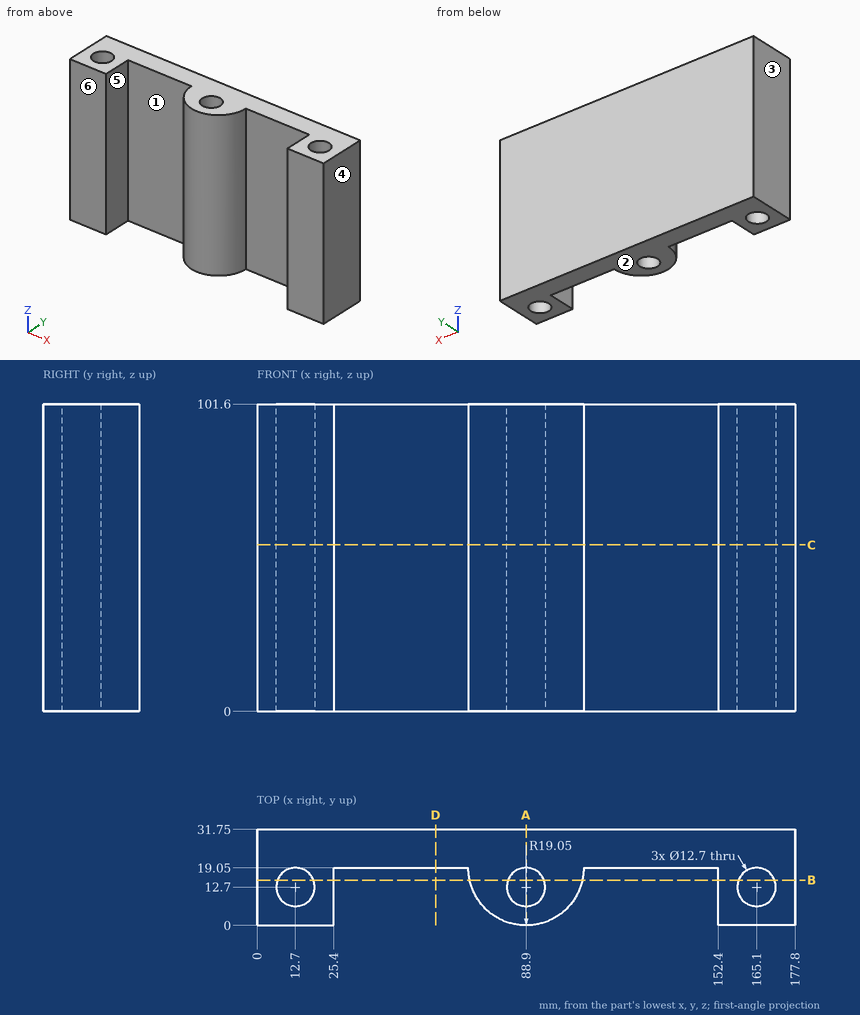
Source: three-view drawing plus pictorial views. Frame: mm from the lowest corner of the part. A direction names the side the tool comes from. Coordinates: 2 decimals unless noted, no trailing zeros. Order: outer loops, then holes, each group sorted by start corner. A loop starts at its lowest first (then second) coordinate and runs counter-clockwise, first axis right, second up. Notation, with made-up numbers: M 67.25,-34 L 100.25,-34 A30 ccw 100.25,4 Z; hole C 31.25,81 d2. An arc over 180 degrees is marked long. One line per question, with ' | ' between items.
Item 1: Section A-A (x = 88.9). Output: boundary loops of the cut face in (y, z).
Geometry results:
outline: M 0,0 L 6.35,0 L 6.35,101.6 L 0,101.6 Z; M 19.05,0 L 31.75,0 L 31.75,101.6 L 19.05,101.6 Z
Item 2: Ray query, line 1 along Y through (x, z) = (12.7, 45); line 2 along X through (y, z) = (7.5, 95); line 3 along X through (y, z) = (13, 68.5). Return the intervals inside material, ascending.
Geometry results:
line 1: y = 0 to 6.35, 19.05 to 31.75 | line 2: x = 0 to 9.06, 16.34 to 25.4, 73.75 to 85.26, 92.54 to 104.05, 152.4 to 161.46, 168.74 to 177.8 | line 3: x = 0 to 6.36, 19.04 to 25.4, 70.84 to 82.56, 95.24 to 106.96, 152.4 to 158.76, 171.44 to 177.8
Item 3: Reachability of the marked faces 1 and 2 from +Z, -Z, +X, -X, +Y, -Y: full face, straight path, thin tool, end or side. Return the list, or none.
Geometry results:
face 1: +Z, -Z, -Y | face 2: -Z, +X, -X, +Y, -Y
Item 4: Pin query (flat end, axial travel): pin 1 (4 mm diameter, centred on y = 16, z = 15, fed in from -X); pin 2 (10 mm diameter, centred on x = 38.5, z = 36.5, fed in from -Y). Return the tip coordinate at first contact, or that it passes through.
Geometry results:
pin 1: stops at x = 0 | pin 2: stops at y = 19.05
Item 5: Section D-D (x = 59). Output: boundary loops of the cut face in (y, z), then the cut area to 3 significant figures.
Geometry results:
outline: M 19.05,0 L 31.75,0 L 31.75,101.6 L 19.05,101.6 Z | area: 1,290 mm^2
Item 6: Draft query along X for the marked faces 3, 4, 5 and 6. Return one class per face: released by +X, released by -X, zero draft, split by the parting line, or undercut.
Geometry results:
face 3: released by -X | face 4: released by +X | face 5: undercut | face 6: zero draft
Item 7: Section C-C (z = 55). Output: boundary loops of the cut face in (x, y), then the cut area to 3 significant figures.
Geometry results:
outline: M 0,0 L 25.4,0 L 25.4,19.05 L 69.85,19.05 A19.05 ccw 107.95,19.05 L 152.4,19.05 L 152.4,0 L 177.8,0 L 177.8,31.75 L 0,31.75 Z; hole C 12.7,12.7 d12.7; hole C 88.9,12.7 d12.7; hole C 165.1,12.7 d12.7 | area: 3,420 mm^2
Item 8: Section B-B (y = 15). Output: boundary loops of the cut face in (x, z), then the cut area to 3 significant figures.
Geometry results:
outline: M 0,0 L 6.78,0 L 6.78,101.6 L 0,101.6 Z; M 18.62,0 L 25.4,0 L 25.4,101.6 L 18.62,101.6 Z; M 70.29,0 L 82.98,0 L 82.98,101.6 L 70.29,101.6 Z; M 94.82,0 L 107.51,0 L 107.51,101.6 L 94.82,101.6 Z; M 152.4,0 L 159.18,0 L 159.18,101.6 L 152.4,101.6 Z; M 171.02,0 L 177.8,0 L 177.8,101.6 L 171.02,101.6 Z | area: 5,340 mm^2
